Read the model definition and answer for the solid it produces. Units are mm, in the model's axes. A direction names the side the tool comes from. Coordinates: 2 decimals unless noted, no trailing zeros. Order: outer loops, then holes, each group sorted by start corner. A loop starts at its lowest first (then second) coordinate and runs counter-clockwise, first axis right, second up. Notation, with made-up numbers: M -38.75,57.25 L -14.75,57.25 A26 ccw -14.75,81.25 Z; hole C 26,1 d9. An arc over 180 degrees is marked long. Put each result on its own line as item: value.
from build123d import *

# Parameters (mm, degrees)
BOSS_EXTRUDE1_DEPTH = 1.5
CUT_EXTRUDE14_DEPTH = 0.4
MIRROR1_OUTLINE_R   = 1.15
MIRROR1_DEPTH       = 0.5099999
MIRROR1_START       = 0.4
MIRROR1_2_DEPTH     = 1.1
MIRROR1_START_2     = 0.5099999
MIRROR1_3_DEPTH     = 0.9900001
SKETCH3_W           = 5.1
SKETCH3_H           = 5.1
CUT_EXTRUDE9_DEPTH  = 28.99107001
SKETCH3_8_W         = 1
SKETCH3_8_H         = 0.6
CUT_EXTRUDE13_DEPTH = 0.4
SKETCH3_5_W         = 13.9
SKETCH3_5_H         = 1.2
CUT_EXTRUDE10_DEPTH = 0.3
LID_OUTLINE_W       = 5.1
LID_OUTLINE_H       = 5.1
LID_DEPTH           = 2
LID_2_OUTLINE_W     = 10.15
LID_2_OUTLINE_H     = 1.2
LID_2_DEPTH         = 0.3
LID_START           = 0.3
LID_3_OUTLINE_W     = 1
LID_3_OUTLINE_H     = 1.2
LID_3_DEPTH         = 0.1


with BuildPart() as part:
    # Sketch1 → Boss-Extrude1 (new body)
    with BuildSketch(Plane(origin=(0, 0, 0), x_dir=(1, 0, 0), z_dir=(0, 1, 0))):
        with BuildLine():
            Line((0, 0), (25, 0))
            Line((25, 0), (25, 11.5))
            ThreePointArc((25, 11.5), (24.707106781, 12.207106781), (24, 12.5))
            Line((24, 12.5), (0, 12.5))
            Line((0, 12.5), (0, 0))
        make_face()
    extrude(amount=BOSS_EXTRUDE1_DEPTH)

    # Sketch1<11> → Cut-Extrude14 (cut)
    with BuildSketch(Plane(origin=(0, 0, 0), x_dir=(1, 0, 0), z_dir=(0, 1, 0))):
        with BuildLine():
            Line((0, 3.75), (0, 0))
            Line((0, 0), (3.75, 0))
            Line((3.75, 0), (3.75, 2.75))
            ThreePointArc((3.75, 2.75), (3.457106781, 3.457106781), (2.75, 3.75))
            Line((2.75, 3.75), (0, 3.75))
        make_face()
    extrude(amount=CUT_EXTRUDE14_DEPTH, mode=Mode.SUBTRACT)

    # Sketch11 → CSK for M2 Countersunk Flat Head Screw1 (revolve, cut)
    with BuildSketch(Plane(origin=(21.5, 1.5, -9), x_dir=(0, 0, 1), z_dir=(1, 0, 0))):
        Polygon((0, 0), (0, 1.5), (1.15, 1.5), (1.15, 0.99), (2.14, 0), align=None)
    revolve(axis=Axis((21.5, 7.85, -9), (0, -1, 0)), mode=Mode.SUBTRACT)

    # Mirror1: read off the stored shape, not the designer's step
    # Mirror1 outline → Mirror1 (add)
    with BuildSketch(Plane(origin=(0, 0, 0), x_dir=(1, 0, 0), z_dir=(0, 1, 0))):
        with BuildLine():
            Line((25, -11.5), (25, 0))
            Line((25, 0), (3.75, 0))
            Line((3.75, 0), (3.75, -2.75))
            ThreePointArc((3.75, -2.75), (3.457106781, -3.457106781), (2.75, -3.75))
            Line((2.75, -3.75), (-2.75, -3.75))
            ThreePointArc((-2.75, -3.75), (-3.457106781, -3.457106781), (-3.75, -2.75))
            Line((-3.75, -2.75), (-3.75, 2.75))
            ThreePointArc((-3.75, 2.75), (-3.457106781, 3.457106781), (-2.75, 3.75))
            Line((-2.75, 3.75), (0, 3.75))
            Line((0, 3.75), (0, 12.5))
            Line((0, 12.5), (-24, 12.5))
            ThreePointArc((-24, 12.5), (-24.707106781, 12.207106781), (-25, 11.5))
            Line((-25, 11.5), (-25, -11.5))
            ThreePointArc((-25, -11.5), (-24.707106781, -12.207106781), (-24, -12.5))
            Line((-24, -12.5), (24, -12.5))
            ThreePointArc((24, -12.5), (24.707106781, -12.207106781), (25, -11.5))
        make_face()
        with Locations((-21.5, -9)):
            Circle(MIRROR1_OUTLINE_R, mode=Mode.SUBTRACT)
        with Locations((21.5, -9)):
            Circle(MIRROR1_OUTLINE_R, mode=Mode.SUBTRACT)
        with Locations((-21.5, 9)):
            Circle(MIRROR1_OUTLINE_R, mode=Mode.SUBTRACT)
    extrude(amount=MIRROR1_DEPTH)

    # Mirror1 2 outline → Mirror1 2 (add)
    with BuildSketch(Plane(origin=(0, 0, 0), x_dir=(1, 0, 0), z_dir=(0, 1, 0)).offset(MIRROR1_START)):
        with BuildLine():
            Line((3.75, -2.75), (3.75, 0))
            Line((3.75, 0), (0, 0))
            Line((0, 0), (0, 3.75))
            Line((0, 3.75), (-2.75, 3.75))
            ThreePointArc((-2.75, 3.75), (-3.457106781, 3.457106781), (-3.75, 2.75))
            Line((-3.75, 2.75), (-3.75, -2.75))
            ThreePointArc((-3.75, -2.75), (-3.457106781, -3.457106781), (-2.75, -3.75))
            Line((-2.75, -3.75), (2.75, -3.75))
            ThreePointArc((2.75, -3.75), (3.457106781, -3.457106781), (3.75, -2.75))
        make_face()
    extrude(amount=MIRROR1_2_DEPTH)

    # Mirror1 3 outline → Mirror1 3 (add)
    with BuildSketch(Plane(origin=(0, 0, 0), x_dir=(1, 0, 0), z_dir=(0, 1, 0)).offset(MIRROR1_START_2)):
        with BuildLine():
            Line((25, -11.5), (25, 0))
            Line((25, 0), (3.75, 0))
            Line((3.75, 0), (3.75, -2.75))
            ThreePointArc((3.75, -2.75), (3.457106781, -3.457106781), (2.75, -3.75))
            Line((2.75, -3.75), (-2.75, -3.75))
            ThreePointArc((-2.75, -3.75), (-3.457106781, -3.457106781), (-3.75, -2.75))
            Line((-3.75, -2.75), (-3.75, 2.75))
            ThreePointArc((-3.75, 2.75), (-3.457106781, 3.457106781), (-2.75, 3.75))
            Line((-2.75, 3.75), (0, 3.75))
            Line((0, 3.75), (0, 12.5))
            Line((0, 12.5), (-24, 12.5))
            ThreePointArc((-24, 12.5), (-24.707106781, 12.207106781), (-25, 11.5))
            Line((-25, 11.5), (-25, -11.5))
            ThreePointArc((-25, -11.5), (-24.707106781, -12.207106781), (-24, -12.5))
            Line((-24, -12.5), (24, -12.5))
            ThreePointArc((24, -12.5), (24.707106781, -12.207106781), (25, -11.5))
        make_face()
    extrude(amount=MIRROR1_3_DEPTH)

    # Mirror1 4: loft between two sections, ruled curve by curve
    mirror1_4_from = [
        Edge.make_three_point_arc((-21.5, 0.51, -7.85), (-20.35, 0.51, -9), (-21.5, 0.51, -10.15)),
        Edge.make_three_point_arc((-21.5, 0.51, -10.15), (-22.65, 0.51, -9), (-21.5, 0.51, -7.85)),
    ]
    mirror1_4_to = [
        Edge.make_three_point_arc((-21.5, 1.5, -6.86), (-19.36, 1.5, -9), (-21.5, 1.5, -11.14)),
        Edge.make_three_point_arc((-21.5, 1.5, -11.14), (-23.64, 1.5, -9), (-21.5, 1.5, -6.86)),
    ]
    mirror1_4 = Solid(Shell([*[Face.make_surface_from_curves(mirror1_4_from[k], mirror1_4_to[k]) for k in range(2)], Face(Wire(mirror1_4_from)), Face(Wire(mirror1_4_to))]))
    add(mirror1_4, mode=Mode.SUBTRACT)

    # Mirror1 5: loft between two sections, ruled curve by curve
    mirror1_5_from = [
        Edge.make_three_point_arc((21.5, 0.51, 7.85), (20.35, 0.51, 9), (21.5, 0.51, 10.15)),
        Edge.make_three_point_arc((21.5, 0.51, 10.15), (22.65, 0.51, 9), (21.5, 0.51, 7.85)),
    ]
    mirror1_5_to = [
        Edge.make_three_point_arc((21.5, 1.5, 6.86), (19.36, 1.5, 9), (21.5, 1.5, 11.14)),
        Edge.make_three_point_arc((21.5, 1.5, 11.14), (23.64, 1.5, 9), (21.5, 1.5, 6.86)),
    ]
    mirror1_5 = Solid(Shell([*[Face.make_surface_from_curves(mirror1_5_from[k], mirror1_5_to[k]) for k in range(2)], Face(Wire(mirror1_5_from)), Face(Wire(mirror1_5_to))]))
    add(mirror1_5, mode=Mode.SUBTRACT)

    # Mirror1 6: loft between two sections, ruled curve by curve
    mirror1_6_from = [
        Edge.make_three_point_arc((-21.5, 0.51, 7.85), (-22.65, 0.51, 9), (-21.5, 0.51, 10.15)),
        Edge.make_three_point_arc((-21.5, 0.51, 10.15), (-20.35, 0.51, 9), (-21.5, 0.51, 7.85)),
    ]
    mirror1_6_to = [
        Edge.make_three_point_arc((-21.5, 1.5, 6.86), (-23.64, 1.5, 9), (-21.5, 1.5, 11.14)),
        Edge.make_three_point_arc((-21.5, 1.5, 11.14), (-19.36, 1.5, 9), (-21.5, 1.5, 6.86)),
    ]
    mirror1_6 = Solid(Shell([*[Face.make_surface_from_curves(mirror1_6_from[k], mirror1_6_to[k]) for k in range(2)], Face(Wire(mirror1_6_from)), Face(Wire(mirror1_6_to))]))
    add(mirror1_6, mode=Mode.SUBTRACT)

    # Sketch3 → Cut-Extrude9 (cut, through all)
    with BuildSketch(Plane.XZ):
        with Locations((16.45, 0)):
            Rectangle(SKETCH3_W, SKETCH3_H)
    extrude(amount=-CUT_EXTRUDE9_DEPTH, mode=Mode.SUBTRACT)

    # Sketch3<8> → Cut-Extrude13 (cut)
    with BuildSketch(Plane.XZ):
        with Locations((13.4, -0.3)):
            Rectangle(SKETCH3_8_W, SKETCH3_8_H)
        with Locations((13.4, 0.3)):
            Rectangle(SKETCH3_8_W, SKETCH3_8_H)
    extrude(amount=-CUT_EXTRUDE13_DEPTH, mode=Mode.SUBTRACT)

    # Sketch3<5> → Cut-Extrude10 (cut)
    with BuildSketch(Plane.XZ):
        with Locations((6.95, 0)):
            Rectangle(SKETCH3_5_W, SKETCH3_5_H)
    extrude(amount=-CUT_EXTRUDE10_DEPTH, mode=Mode.SUBTRACT)

    # lid: read off the stored shape, not the designer's step
    # lid outline → lid (cut)
    with BuildSketch(Plane(origin=(0, 0, 0), x_dir=(1, 0, 0), z_dir=(0, 1, 0))):
        with Locations((-16.45, 0)):
            Rectangle(LID_OUTLINE_W, LID_OUTLINE_H)
    extrude(amount=LID_DEPTH, mode=Mode.SUBTRACT)

    # lid 2 outline → lid 2 (cut)
    with BuildSketch(Plane(origin=(0, 0, 0), x_dir=(1, 0, 0), z_dir=(0, 1, 0))):
        with Locations((-8.825, 0)):
            Rectangle(LID_2_OUTLINE_W, LID_2_OUTLINE_H)
    extrude(amount=LID_2_DEPTH, mode=Mode.SUBTRACT)

    # lid 3 outline → lid 3 (cut)
    with BuildSketch(Plane(origin=(0, 0, 0), x_dir=(1, 0, 0), z_dir=(0, 1, 0)).offset(LID_START)):
        with Locations((-13.4, 0)):
            Rectangle(LID_3_OUTLINE_W, LID_3_OUTLINE_H)
    extrude(amount=LID_3_DEPTH, mode=Mode.SUBTRACT)


solid = part.part
Q1. Given pin 1 (1.4 mm diameter, centred on x = -21.5, z = 9, fed in from +Y); pin 2 (3.5 mm diameter, centred on x = -21.5, z = -9, fed in from +Y), each flat-ended and moving along its own axis, determine where each tip first touches the part or whether it passes through.
Answers below:
pin 1: passes through
pin 2: stops at y = 1.11
Q2. For a pull along Z with two mould halves and no side action, classify faces 4 (the face through (0, 1, -12.5)), 5 (the face through (21.94, 0.259, -7.938)), 6 (the face through (-25, 1, 0)), 7 (the face through (16, 1, -2.55)) as +Z half, -Z half, draft (parallel to the pull), parting line (faces both ways), or undercut.
Answers below:
face 4: -Z half
face 5: undercut
face 6: draft
face 7: undercut
Q3. Find section B-B on z = 1.75. Write down the section's boundary in (x, y).
Answers below:
outline: M -25,0 L -19,0 L -19,1.5 L -25,1.5 Z; M -13.9,0 L -3.75,0 L -3.75,0.4 L 3.75,0.4 L 3.75,0 L 13.9,0 L 13.9,1.5 L -13.9,1.5 Z; M 19,0 L 25,0 L 25,1.5 L 19,1.5 Z
Q4. Consider line 1 along Z through (x, y) = (21.5, 0.15); line 2 along X through (y, z) = (0.3, 9); line 3 along X through (y, z) = (0.45, 0). Determine where each line is inside the solid, lowest interval first.
Answers below:
line 1: z = -12.5 to -10.15, -7.85 to 7.85, 10.15 to 12.5
line 2: x = -25 to -22.65, -20.35 to 20.35, 22.65 to 25
line 3: x = -25 to -19, -13.9 to 13.9, 19 to 25
Q5. Find section C-C on z = 9. Give the number of separate pieces and of enclosed holes in the cut face, plus the area to 3 significant figures.
Answers below:
separate pieces: 3
enclosed holes: 0
area: 66.1 mm^2
Q6. A tool of negligible diameter and unlimited length cuts with its end or side. For faces 1 (the face through (-3.449, 0.197, 3.465)), 2 (the face through (25, 1, 0)), 3 (the face through (13.9, 1, 0)), from which of +Z, -Z, +X, -X, +Y, -Y can it reach the whole face along a straight path? Write none if from no direction.
Answers below:
face 1: -Y
face 2: +Z, -Z, +X, +Y, -Y
face 3: +Y, -Y
Q7. Find section A-A on x = -17. Write down the section's boundary in (y, z).
Answers below:
outline: M 0,-12.5 L 1.5,-12.5 L 1.5,-2.55 L 0,-2.55 Z; M 0,2.55 L 1.5,2.55 L 1.5,12.5 L 0,12.5 Z
